```python
from build123d import *

# Parameters (mm, degrees)
ESQUISSE3_R             = 13.9
ESQUISSE3_R_2           = 1.8
BOSS_EXTRU_1_DEPTH      = 6
ESQUISSE5_R             = 6
BOSS_EXTRU_2_DEPTH      = 15
ENL_V_MAT_EXTRU_2_DEPTH = 11.8
BOSS_EXTRU_3_REACH      = 37.097
BOSS_EXTRU_3_END_RADIUS = 13.9
BOSS_EXTRU_3_START      = -3
ESQUISSE7_W             = 10
ESQUISSE7_H             = 15
ESQUISSE11_R            = 2.2
ENL_V_MAT_EXTRU_3_DEPTH = 14
ENL_V_START             = -5
ENL_V_MAT_EXTRU_4_DEPTH = 3.5


with BuildPart() as part:
    # Esquisse3 → Boss.-Extru.1 (new body)
    with BuildSketch(Plane(origin=(0, 0, 0), x_dir=(1, 0, 0), z_dir=(0, 1, 0))):
        with Locations(Location((0, 0, 0), (0, 0, 270))):
            Circle(ESQUISSE3_R)
        with Locations(Location((0, 10.5, 0), (0, 0, 270))):
            Circle(ESQUISSE3_R_2, mode=Mode.SUBTRACT)
        with Locations(Location((9.09326674, 5.25, 0), (0, 0, 270))):
            Circle(ESQUISSE3_R_2, mode=Mode.SUBTRACT)
        with Locations(Location((9.09326674, -5.25, 0), (0, 0, 270))):
            Circle(ESQUISSE3_R_2, mode=Mode.SUBTRACT)
        with Locations(Location((0, -10.5, 0), (0, 0, 270))):
            Circle(ESQUISSE3_R_2, mode=Mode.SUBTRACT)
        with Locations(Location((-9.09326674, -5.25, 0), (0, 0, 270))):
            Circle(ESQUISSE3_R_2, mode=Mode.SUBTRACT)
        with Locations(Location((-9.09326674, 5.25, 0), (0, 0, 270))):
            Circle(ESQUISSE3_R_2, mode=Mode.SUBTRACT)
    extrude(amount=BOSS_EXTRU_1_DEPTH)

    # Esquisse5 → Boss.-Extru.2 (add)
    with BuildSketch(Plane(origin=(0, 6, 0), x_dir=(1, 0, 0), z_dir=(0, 1, 0))):
        with Locations(Location((0, 0, 0), (0, 0, 270))):
            Circle(ESQUISSE5_R)
    extrude(amount=BOSS_EXTRU_2_DEPTH)

    # Esquisse6 → Enlèv. mat.-Extru.2 (cut)
    with BuildSketch(Plane(origin=(0, 21, 0), x_dir=(1, 0, 0), z_dir=(0, 1, 0))):
        with BuildLine():
            Line((-1.897366596, 2.7), (1.897366596, 2.7))
            ThreePointArc((1.897366596, 2.7), (0, -3.3), (-1.897366596, 2.7))
        make_face()
    extrude(amount=-ENL_V_MAT_EXTRU_2_DEPTH, mode=Mode.SUBTRACT)

    # Boss.-Extru.3: up to this cylinder (the profile starts inside it)
    boss_extru_3_end = Plane(origin=(0, 13.5, 0), z_dir=(0, -1, 0)) * Cylinder(BOSS_EXTRU_3_END_RADIUS, 102.994, mode=Mode.PRIVATE)
    # Esquisse7 → Boss.-Extru.3 (add, up to the surface)
    with BuildSketch(Plane(origin=(0, 0, -6), x_dir=(-1, 0, 0), z_dir=(0, 0, -1)).offset(BOSS_EXTRU_3_START), mode=Mode.PRIVATE) as boss_extru_3_sk1:
        with Locations((0, 13.5)):
            Rectangle(ESQUISSE7_W, ESQUISSE7_H)
    boss_extru_3_tool1 = extrude(boss_extru_3_sk1.sketch, amount=BOSS_EXTRU_3_REACH, mode=Mode.PRIVATE) & boss_extru_3_end
    add(boss_extru_3_tool1.solids().sort_by_distance((0, 13.5, -3))[0])

    # Esquisse11 → Enlèv. mat.-Extru.3 (cut)
    with BuildSketch(Plane(origin=(0, 0, -13.9), x_dir=(-1, 0, 0), z_dir=(0, 0, -1))):
        with Locations(Location((0, 12.707359669, 0), (0, 0, 329.591587588))):
            Circle(ESQUISSE11_R)
    extrude(amount=-ENL_V_MAT_EXTRU_3_DEPTH, mode=Mode.SUBTRACT)

    # Esquisse12 → Enlèv. mat.-Extru.4 (cut)
    with BuildSketch(Plane(origin=(0, 0, -13.9), x_dir=(-1, 0, 0), z_dir=(0, 0, -1)).offset(ENL_V_START)):
        Polygon((0, 16.357656746), (-2.1075, 16.357656746), (-4.215, 12.707359669), (-2.1075, 9.057062592), (2.1075, 9.057062592), (5, 9.057062592), (5, 16.357656746), align=None)
    extrude(amount=-ENL_V_MAT_EXTRU_4_DEPTH, mode=Mode.SUBTRACT)


solid = part.part
```
For this review, take the finished solid that the model builds, in its own axes (mm). A direction names the side the tool comes from. Coordinates: 2 decimals unless noted, no trailing zeros. Loops run counter-clockwise (first coordinate to the right, second up) from the corner with the lowest first, then second, coordinate; pieces in that order, holes last.
1. Add section B-B, the plane z = -5. Give the boundary of the cut face in (x, y), then the cut area to 3 significant figures.
2. Mouldability with a two-part tool opening along Z and no side actions: class faces 6 (the flat face through (0.2, 6, 6.2)), 7 (the cylindrical face through (0.08, 2.96, -12.3)), 8 (the cylindrical face through (0, 13, 6)) as +Z half, -Z half, draft (parallel to the pull), parting line (faces both ways), or undercut.
3. Add section A-A, the plane x = 0. Count the separate pieces of the cut face and the enclosed holes in it, then the cut area to 3 significant figures.
4. Add section C-C, the plane y = 18.5. Give the boundary of the cut face in (x, z), then the cut area to 3 significant figures.
5. Insertion check: P1, Ø12, axis at x = 5, y = 16, coming from the +Z side; P2, Ø5, axis at y = 15.5, z = -8, coming from the +X side; P3, Ø5, axis at x = 0, z = 0.5, coming from the +Y side; P4, Ø3, axis at x = 9.09, z = 5.25, coming from the -Y side. Each pin has a flat end and moves straight along its axis. Give the tip position at first contact, or say it passes through.
6. Add section D-D, the plane z = 11.25. Give the boundary of the cut face in (x, y).
7. For line 1 (Z direction, x = 7.5, y = 4.5); line 2 (Z direction, x = -2.5, y = 11.5); line 3 (X direction, y = 2.1, z = 5.25), list the stretches that pass through material, from the lowest coordinate up.
8. For faces 1 (the flat face through (0, 0, 0)), 2 (the flat face through (0, 10, -2.7)), 3 (the flat face through (-1, 9.057, -7)), 4 (the cylindrical face through (0.11, 10.51, -11.44)), 5 (the flat face through (-5, 13.4, -9.1)), list the 3-axis set-ups (+Z, -Z, +X, -X, +Y, -Y) from which the entire face can be reached by the end or side of a thin tool; tool diameter is ignored.
Result:
1. outline: (-12.97, 0) - (-10.88, 0) - (-10.88, 6) - (-12.97, 6) - close; (-7.31, 0) - (7.31, 0) - (7.31, 6) - (5, 6) - (5, 21) - (-5, 21) - (-5, 6) - (-7.31, 6) - close; (10.88, 0) - (12.97, 0) - (12.97, 6) - (10.88, 6) - close; hole circle Ø4.4 at (0, 12.71)
1. area: 248 mm2
2. face 6: draft
2. face 7: undercut
2. face 8: parting line
3. separate pieces: 3
3. enclosed holes: 0
3. area: 292 mm2
4. outline: (-5, -12.97) arc R13.9 ccw to (5, -12.97) - (5, -3.32) arc R6 ccw (long way) to (-5, -3.32) - close; hole (-1.9, -2.7) - (1.9, -2.7) arc R3.3 ccw (long way) to start
4. area: 164 mm2
5. P1: stops at z = 6
5. P2: stops at x = 5
5. P3: stops at y = 9.2
5. P4: passes through
6. outline: (-8.16, 0) - (-1.64, 0) - (-1.64, 6) - (-8.16, 6) - close; (1.64, 0) - (8.16, 0) - (8.16, 6) - (1.64, 6) - close
7. line 1: z = -11.7 to -6.09, -4.41 to 4.41, 6.09 to 11.7
7. line 2: z = -13.67 to -8.9, -5.4 to -2.15, 2.15 to 5.45
7. line 3: x = -12.87 to -10.89, -7.29 to 7.29, 10.89 to 12.87
8. face 1: +Z, -Z, +X, -X, -Y
8. face 2: +Y
8. face 3: -X
8. face 4: -Z
8. face 5: -Z, -X, +Y
